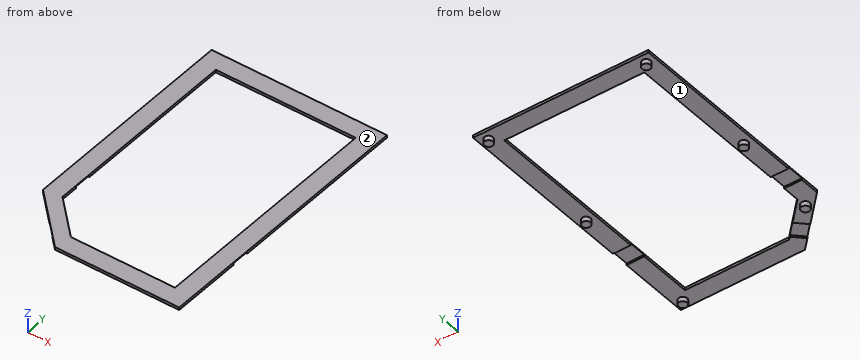
Autodesk Inventor part; units mm, degrees
ref_plane "YZ Plane" through (0, 0, 0) normal (1, 0, 0) x (0, 1, 0)
ref_plane "XZ Plane" through (0, 0, 0) normal (0, 1, 0) x (-1, 0, 0)
ref_plane "XY Plane" through (0, 0, 0) normal (0, 0, 1) x (1, 0, 0)
sketch "Skizze1" plane through (0, 0, 0) normal (0, 0, 1) x (1, 0, 0)
  line L0 (49.5001, 297.0913) -> (-49.5001, 297.0913)
  line L1 (49.5001, 143.8903) -> (49.5001, 297.0913)
  line L2 (-49.5001, 297.0913) -> (-49.5001, 143.8903) construction
  line L3 (-49.5001, 143.8903) -> (49.5001, 143.8903) construction
  circle A0 centre (-29.7001, 148.7389) radius 1.75 construction
  circle A1 centre (-44.8001, 148.7389) radius 1.75 construction
  circle A2 centre (-24.6237, 162.7718) radius 1.75 construction
  circle A3 centre (-20.9666, 159.2418) radius 1.75 construction
  circle A4 centre (44.5001, 148.8903) radius 2.5 construction
  circle A5 centre (44.5001, 220.1498) radius 2.5 construction
  circle A6 centre (-44.5001, 220.1498) radius 2.5 construction
  circle A7 centre (-44.5001, 292.0913) radius 2.5 construction
  circle A8 centre (44.5001, 292.0913) radius 2.5 construction
  line L4 (49.5001, 143.8903) -> (-20.6089, 143.8903)
  line L5 (-20.6089, 143.8903) -> (-49.5001, 172.7815)
  line L6 (-49.5001, 172.7815) -> (-49.5001, 297.0913)
  line L7 (-39.5001, 287.0913) -> (39.5001, 287.0913)
  line L8 (39.5001, 287.0913) -> (39.5001, 153.8903)
  line L9 (39.5001, 153.8903) -> (-19.2952, 153.8903)
  line L10 (-19.2952, 153.8903) -> (-39.5001, 174.0952)
  line L11 (-39.5001, 174.0952) -> (-39.5001, 287.0913)
  point P0 (0, 0)
  dimension "d0" = 135
  dimension "d1" = 8
  dimension "d2" = 3
  dimension "d3" = 10
  dimension "d4" = 10
  dimension "d5" = 10
  dimension "d6" = 10
extrude "Extrusion1" add sketch "Skizze1" along normal blind 1.5
sketch "Skizze2" plane through (0, 0, 0) normal (0, 0, -1) x (-1, 0, 0)
  circle A0 centre (44.5001, 220.1498) radius 2.4
  circle A1 centre (44.5001, 292.0913) radius 2.4
  circle A2 centre (-44.5001, 292.0913) radius 2.4
  circle A3 centre (-44.5001, 220.1498) radius 2.4
  circle A4 centre (-44.5001, 148.8903) radius 2.4
  circle A5 centre (40.1569, 169.0952) radius 2.5 construction
  circle A6 centre (40.1569, 169.0952) radius 2.4
  point P0 (0, 0)
  dimension "d19" = 4.8
  dimension "d20" = 4.8
extrude "Extrusion2" add sketch "Skizze2" along normal blind 2.6
sketch "Skizze3" plane through (0, 0, 0) normal (0, 0, -1) x (-1, 0, 0)
  line L0 (-49.5001, 143.8903) -> (-49.5001, 297.0913)
  line L1 (-39.5001, 287.0913) -> (-39.5001, 153.8903)
  line L2 (-49.5001, 183.8903) -> (-39.5001, 183.8903)
  line L3 (-39.5001, 183.8903) -> (-39.5001, 193.8903)
  line L4 (-39.5001, 193.8903) -> (-49.5001, 193.8903)
  line L5 (-49.5001, 193.8903) -> (-49.5001, 183.8903)
  line L6 (39.5001, 287.0913) -> (39.5001, 174.0952)
  line L7 (49.5001, 297.0913) -> (49.5001, 172.7815)
  line L8 (39.5001, 183.8903) -> (49.5001, 183.8903)
  line L9 (49.5001, 183.8903) -> (49.5001, 193.8903)
  line L10 (49.5001, 193.8903) -> (39.5001, 193.8903)
  line L11 (39.5001, 193.8903) -> (39.5001, 183.8903)
  line L12 (39.5001, 174.0952) -> (19.2952, 153.8903)
  line L13 (20.7094, 155.3045) -> (26.3662, 149.6477)
  line L14 (49.5001, 172.7815) -> (20.6089, 143.8903)
  line L15 (26.3662, 149.6477) -> (33.4373, 156.7188)
  line L16 (33.4373, 156.7188) -> (27.7805, 162.3756)
  line L17 (27.7805, 162.3756) -> (20.7094, 155.3045)
  line L18 (20.6089, 143.8903) -> (-49.5001, 143.8903)
  point P0 (0, 0)
  dimension "d11" = 10
  dimension "d12" = 10
  dimension "d13" = 10
  dimension "d14" = 0
  dimension "d15" = 40
  dimension "d16" = 2
extrude "Extrusion3" cut sketch "Skizze3" against normal blind 1 contours L0 L4 L1 L2 | L13 L12 L16 L14 | L8 L6 L10 L7
equation "\"d4\" = d3"
equation "\"d5\" = d3"
equation "\"d6\" = d3"
equation "\"d20\" = d19"
equation "\"d12\" = d11"
equation "\"d13\" = d11"
properties part number "Backplate_V2"
Design review of the part built by this model. Coordinates are the model's own, in mm. Face numbers are marked on the shaded views. Coordinates: 2 decimals unless noted, no trailing zeros. Order: outer loops, then holes, each group sorted by start corner. A loop starts at its lowest first (then second) coordinate and runs counter-clockwise, first axis right, second up.
1) Clearance check with flat-ended pins moving along their axes: pin 1 (11 mm diameter, centred on x = -43.5, y = 189.5, fed in from -Z); pin 2 (0.5 mm diameter, centred on x = -43.5, z = 0.5, fed in from -Y); pin 3 (3 mm diameter, centred on x = 43, y = 188, fed in from -Z). State where each tip first meets the part, or that it passes through.
2) Take a section at C-C, the plane z = -1.2. Give the boundary of the cut face in (x, y).
3) Take a section at A-A, the plane y = 253.5. Give the boundary of the cut face in (x, z).
4) Wall thickness on line 1 along Y through (x, z) = (29, 0.15); line 2 along X through (y, z) = (198.5, 1.1); line 3 along Z through (x, y) = (43.5, 233): over which ranges is each line inside the solid? List them lowest first.
5) Mouldability with a two-part tool opening along Y and no side actions: class the marked faces 1 and 2 as +Y half, -Y half, draft (parallel to the pull), parting line (faces both ways), or undercut.
6) Take a section at B-B, the plane x = 18. Give the boundary of the cut face in (y, z), and give its area (3 significant figures).
Returned:
1. pin 1: stops at z = 0
1. pin 2: stops at y = 166.53
1. pin 3: stops at z = 1
2. outline: circle Ø4.8 at (-44.5, 220.15); circle Ø4.8 at (-44.5, 292.09); circle Ø4.8 at (-40.16, 169.1); circle Ø4.8 at (44.5, 148.89); circle Ø4.8 at (44.5, 220.15); circle Ø4.8 at (44.5, 292.09)
3. outline: (-49.5, 0) - (-39.5, 0) - (-39.5, 1.5) - (-49.5, 1.5) - close; (39.5, 0) - (49.5, 0) - (49.5, 1.5) - (39.5, 1.5) - close
4. line 1: y = 143.89 to 153.89, 287.09 to 297.09
4. line 2: x = -49.5 to -39.5, 39.5 to 49.5
4. line 3: z = 0 to 1.5
5. face 1: undercut
5. face 2: draft
6. outline: (143.89, 0) - (153.89, 0) - (153.89, 1.5) - (143.89, 1.5) - close; (287.09, 0) - (297.09, 0) - (297.09, 1.5) - (287.09, 1.5) - close
6. area: 30.0 mm2
